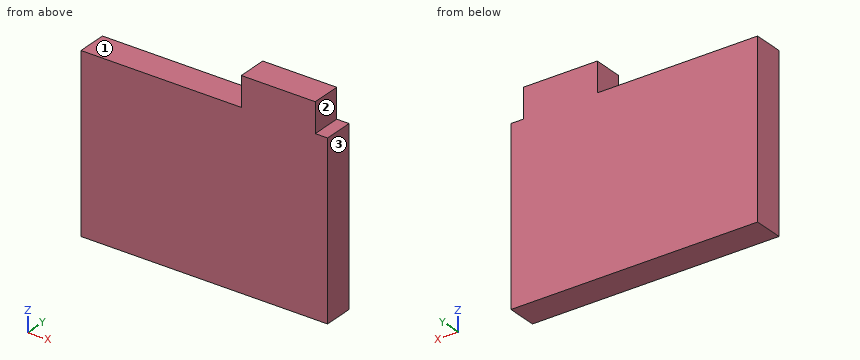
Autodesk Inventor part; units mm, degrees
ref_plane "YZ Plane" through (0, 0, 0) normal (1, 0, 0) x (0, 1, 0)
ref_plane "XZ Plane" through (0, 0, 0) normal (0, 1, 0) x (-1, 0, 0)
ref_plane "XY Plane" through (0, 0, 0) normal (0, 0, 1) x (1, 0, 0)
sketch "Sketch2" plane through (0, 0, 0) normal (0, 1, 0) x (-1, 0, 0)
  line L0 (25, -17.5) -> (-25, -17.5)
  line L1 (-25, -17.5) -> (-25, 17.5)
  line L2 (25, -17.5) -> (-25, 17.5) construction
  line L3 (-25, -17.5) -> (25, 17.5) construction
  line L4 (-22.5, 17.5) -> (-7.5, 17.5)
  line L5 (-7.5, 17.5) -> (-7.5, 23.5)
  line L6 (-7.5, 23.5) -> (-22.5, 23.5)
  line L7 (-22.5, 23.5) -> (-22.5, 17.5)
  line L8 (25, -17.5) -> (25, 17.5)
  line L9 (25, 17.5) -> (-25, 17.5)
  point P0 (0, 0)
  point P1 (0, 0)
  point P2 (-7.5, 17.5)
  dimension "d0" = 50
  dimension "d1" = 35
  dimension "d58" = 2.5
  dimension "d59" = 15
  dimension "d60" = 6
extrude "Extrusion12" add sketch "Sketch2" along normal blind 6
sketch "Sketch7" plane through (0, 6, 0) normal (0, 1, 0) x (1, 0, 0)
  line L0 (25, -17.5) -> (25, 17.5)
  line L1 (-25, -17.5) -> (7.5, -17.5)
  point P0 (0, 0)
extrude "Extrusion13" [suppressed]
properties part number "Pared_caja_reduccion_frontal"
Can you work these out from the model? Positions are in its coordinate system, mm. Face numbers are marked on the shaded views. A direction names the side the tool comes from. Coordinates: 2 decimals unless noted, no trailing zeros. Write each loop counter-clockwise with the first axis right and the second up, starting at its lowest first coordinate (ties: lowest second). Pieces come first, ordered by that corner, then holes. Notation, with made-up numbers: M -6,19 L 27,19 A27 ccw 27,55 Z; hole C 74,3.25 d9. An arc over 180 degrees is marked long. Answer as CSV lines item,"result".
Item 1: Please list where these lines run through material, in increasing order: line 1 along Z through (x, y) = (-3, 0.4); line 2 along X through (y, z) = (1.25, 21.5).
Geometry results:
line 1,"z = -17.5 to 17.5"
line 2,"x = 7.5 to 22.5"
Item 2: On a 3-axis mill with a long thin cutter (end or side, diameter ignored), from which of +Z, -Z, +X, -X, +Y, -Y can I reach the whole of each face in a straight line? I mean the marked faces 1, 2 and 3. Say none if no direction works.
Geometry results:
face 1,"+Z, -X, +Y, -Y"
face 2,"+Z, +X, +Y, -Y"
face 3,"+Z, -Z, +X, +Y, -Y"
Item 3: I'm going to push flat-ended pins straight in: P1, Ø1.5, axis at x = -15.5, z = 19, coming from the +Y side; P2, Ø3, axis at y = 4.5, z = 22, coming from the +X side; P3, Ø3, axis at x = -5, y = 4.5, coming from the +Z side. Where does each tip first touch, or does it pass through?
Geometry results:
P1,"passes through"
P2,"stops at x = 22.5"
P3,"stops at z = 17.5"
Item 4: Imagine slicing it at B-B on x = 4.5. List the corners of the cut face in (y, z) for me.
Geometry results:
outline,"M 0,-17.5 L 6,-17.5 L 6,17.5 L 0,17.5 Z"
Item 5: Imagine slicing it at A-A on y = 3.9. List the corners of the cut face in (x, z) for me.
Geometry results:
outline,"M -25,-17.5 L 25,-17.5 L 25,17.5 L 22.5,17.5 L 22.5,23.5 L 7.5,23.5 L 7.5,17.5 L -25,17.5 Z"
Item 6: Imagine slicing it at C-C on z = 20.5. List the corners of the cut face in (x, y) for me, plus the area to 3 significant figures.
Geometry results:
outline,"M 7.5,0 L 22.5,0 L 22.5,6 L 7.5,6 Z"
area,"90.0 mm2"
